Verification items for the finished model (mm, model axes). Round coordinates to 2 decimals unless told otherwise and drop trailing zeros. Loops run counter-clockwise (first coordinate to the right, second up) from the corner with the lowest first, then second, coordinate; pieces in that order, holes last. Notation, with made-up numbers: (83.5, 29.25) - (112.5, 29.25) arc R17 cw to (112.5, 57.25) - close; hole circle Ø8 at (-30, 68). An arc over 180 degrees is marked (long way). Use a Markdown table: item, result. Add a question column.
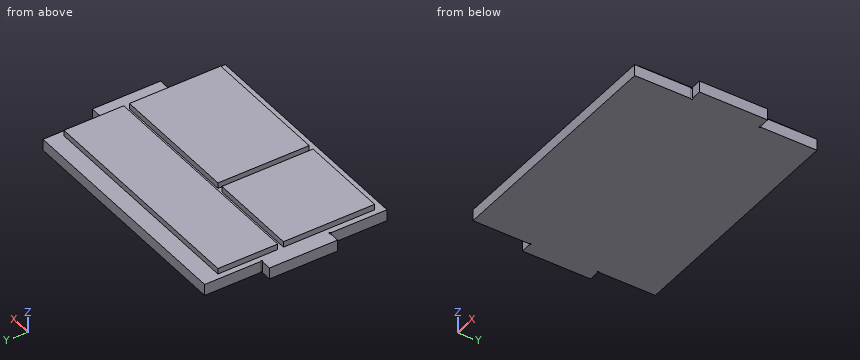
```python
from build123d import *

# Parameters (mm, degrees)
F0_W     = 133.35
F0_H     = 101.6
F1_DEPTH = 6.35
F2_W     = 6.35
F2_H     = 37.973
F3_DEPTH = 6.35
F4_W     = 127
F4_H     = 33.3375
F4_H_2   = 50.8
F5_DEPTH = 3.175
F6_W     = 3.175
F6_H     = 50.8
F7_DEPTH = 3.175
F9_DEPTH = 9.526


with BuildPart() as f1:
    # F0 (on Top) → F1 (new body)
    with BuildSketch(Plane.XY):
        Rectangle(F0_W, F0_H)
    extrude(amount=F1_DEPTH)

    # F2 (on face) → F3 (join)
    with BuildSketch(Plane.XY.offset(6.35)):
        with Locations((-69.85, 0)):
            Rectangle(F2_W, F2_H)
        with Locations((69.85, 0)):
            Rectangle(F2_W, F2_H)
    extrude(amount=-F3_DEPTH)

    # F4 (on face) → F5 (join)
    with BuildSketch(Plane.XY.offset(6.35)):
        with Locations((0, 24.60625)):
            Rectangle(F4_W, F4_H)
        with Locations((0, -20.6375)):
            Rectangle(F4_W, F4_H_2)
    extrude(amount=F5_DEPTH)

    # F6 (on face) → F7 (cut)
    with BuildSketch(Plane.XY.offset(9.525)):
        with Locations((-11.1125, -20.6375)):
            Rectangle(F6_W, F6_H)
    extrude(amount=-F7_DEPTH, mode=Mode.SUBTRACT)

    # F8 (on face) → F9 (cut, through all)
    with BuildSketch(Plane(origin=(0, 0, 0), x_dir=(1, 0, 0), z_dir=(0, 0, -1))):
        with BuildLine():
            ThreePointArc((-67.183, 18.9865), (-66.31579, 18.62729), (-66.675, 19.4945))
            Line((-66.675, 19.4945), (-66.675, 18.9865))
            Line((-66.675, 18.9865), (-67.183, 18.9865))
        make_face()
        with BuildLine():
            Line((-66.675, -18.9865), (-66.675, -19.4945))
            ThreePointArc((-66.675, -19.4945), (-66.31579, -18.62729), (-67.183, -18.9865))
            Line((-67.183, -18.9865), (-66.675, -18.9865))
        make_face()
        with BuildLine():
            ThreePointArc((67.183, -18.9865), (66.31579, -18.62729), (66.675, -19.4945))
            Line((66.675, -19.4945), (66.675, -18.9865))
            Line((66.675, -18.9865), (67.183, -18.9865))
        make_face()
        with BuildLine():
            ThreePointArc((66.675, 19.4945), (66.31579, 18.62729), (67.183, 18.9865))
            Line((67.183, 18.9865), (66.675, 18.9865))
            Line((66.675, 18.9865), (66.675, 19.4945))
        make_face()
        with BuildLine():
            Line((66.675, 18.9865), (66.675, 19.4945))
            ThreePointArc((66.675, 19.4945), (66.31579, 18.62729), (67.183, 18.9865))
            Line((67.183, 18.9865), (66.675, 18.9865))
        make_face()
        with BuildLine():
            Line((66.675, -18.9865), (67.183, -18.9865))
            ThreePointArc((67.183, -18.9865), (66.31579, -18.62729), (66.675, -19.4945))
            Line((66.675, -19.4945), (66.675, -18.9865))
        make_face()
        with BuildLine():
            ThreePointArc((-66.675, -19.4945), (-66.31579, -18.62729), (-67.183, -18.9865))
            Line((-67.183, -18.9865), (-66.675, -18.9865))
            Line((-66.675, -18.9865), (-66.675, -19.4945))
        make_face()
    extrude(amount=-F9_DEPTH, mode=Mode.SUBTRACT)


solid = f1.part
```
Q1. Section check C-C on y = -36.5. Record the cut outline in (x, z) (3 decimals).
Q2. Thickness scan on line 1 along X through (y, z) = (-39.5, 7.5) (3 decimals); line 2 along Y through (x, z) = (57, 7.5) (1 decimal); line 3 along X through (y, z) = (-29, 0.5) (3 decimals). Record the ranges inside material, lowest first.
Q3. Go/stop test with flat-tipped pins: pin 1 Ø0.8 at (x, y) = (66.68, 18.99) entering from +Z; pin 2 Ø5 at (y, z) = (-27, 2) entering from -X (3 decimals); pin 3 Ø2.5 at (y, z) = (-21.5, 8.5) entering from +X; pin 4 Ø1 at (x, z) = (-39.5, 7.5) entering from +Y (3 decimals). Record where each tip stops, or that it passes through.
Q4. Section check A-A on z = 8. Record the cut outline in (x, y) (1 decimal).
Determined:
| question | item | result |
|---|---|---|
| 1 | outline | (-66.675, 0) - (66.675, 0) - (66.675, 6.35) - (63.5, 6.35) - (63.5, 9.525) - (-9.525, 9.525) - (-9.525, 6.35) - (-12.7, 6.35) - (-12.7, 9.525) - (-63.5, 9.525) - (-63.5, 6.35) - (-66.675, 6.35) - close |
| 2 | line 1 | x = -63.5 to -12.7, -9.525 to 63.5 |
| 2 | line 2 | y = -46 to 4.8, 7.9 to 41.3 |
| 2 | line 3 | x = -66.675 to 66.675 |
| 3 | pin 1 | passes through |
| 3 | pin 2 | stops at x = -66.675 |
| 3 | pin 3 | stops at x = 63.5 |
| 3 | pin 4 | stops at y = 41.275 |
| 4 | outline | (-63.5, -46) - (-12.7, -46) - (-12.7, 4.8) - (-63.5, 4.8) - close; (-63.5, 7.9) - (63.5, 7.9) - (63.5, 41.3) - (-63.5, 41.3) - close; (-9.5, -46) - (63.5, -46) - (63.5, 4.8) - (-9.5, 4.8) - close |
